For this review, use the dimensioned drawing (mm, ordinates from the lowest corner) and the shaded views. A direction names the side the tool comes from. Coordinates: 2 decimals unless noted, no trailing zeros. Order: outer loops, then holes, each group sorted by start corner. A loop starts at its lowest first (then second) coordinate and runs counter-clockwise, first axis right, second up. Notation, with made-up numbers: (64, 49) -> (87, 49) arc R17 cw to (87, 79) -> close; hole circle Ø8 at (30, 29.5). An arc over 180 degrees is marked (long way). Return JSON: item names as keys, results as strings. Group by question number.
Item 1: Insertion check: pin 1 (7 mm diameter, centred on y = 2.5, z = 3, fed in from -X); pin 2 (1 mm diameter, centred on x = 6, z = 7.5, fed in from -Y); pin 3 (2 mm diameter, centred on x = 13.5, z = 6.5, fed in from -Y). Each pin has a flat end and moves straight along its axis. Give the tip position at first contact, or say it passes through.
Item 2: Draft analysis for pull direction Y (two halves, no side actions). For the marked faces 1, 2 and 3, state which applies: +Y half, -Y half, draft (parallel to the pull), parting line (faces both ways), or undercut.
Item 3: Take a section at C-C (z = 8.5). Write out the cut boundary in (x, y).
Item 4: Take a section at A-A (x = 2.54). Write out the cut boundary in (y, z) (3 decimals).
Item 5: For line 1 along Z through (x, y) = (2.54, 12.25) (3 decimals); line 2 along Y through (x, z) = (4.5, 11.5); line 3 along Y through (x, z) = (14.25, 6.35) (3 decimals), list the stretches that pass through material, from the lowest coordinate up.
Item 6: Machinability: for the marked faces 4 and 5, which of the approach directions +Z, -Z, +X, -X, +Y, -Y give a long, thin tool a straight path to every point of the face, cutting with its end or side? Answer none if there is none.
Item 7: Take a section at D-D (z = 6.35). Write out the cut boundary in (x, y) (3 decimals), then the cut area to 3 significant figures.
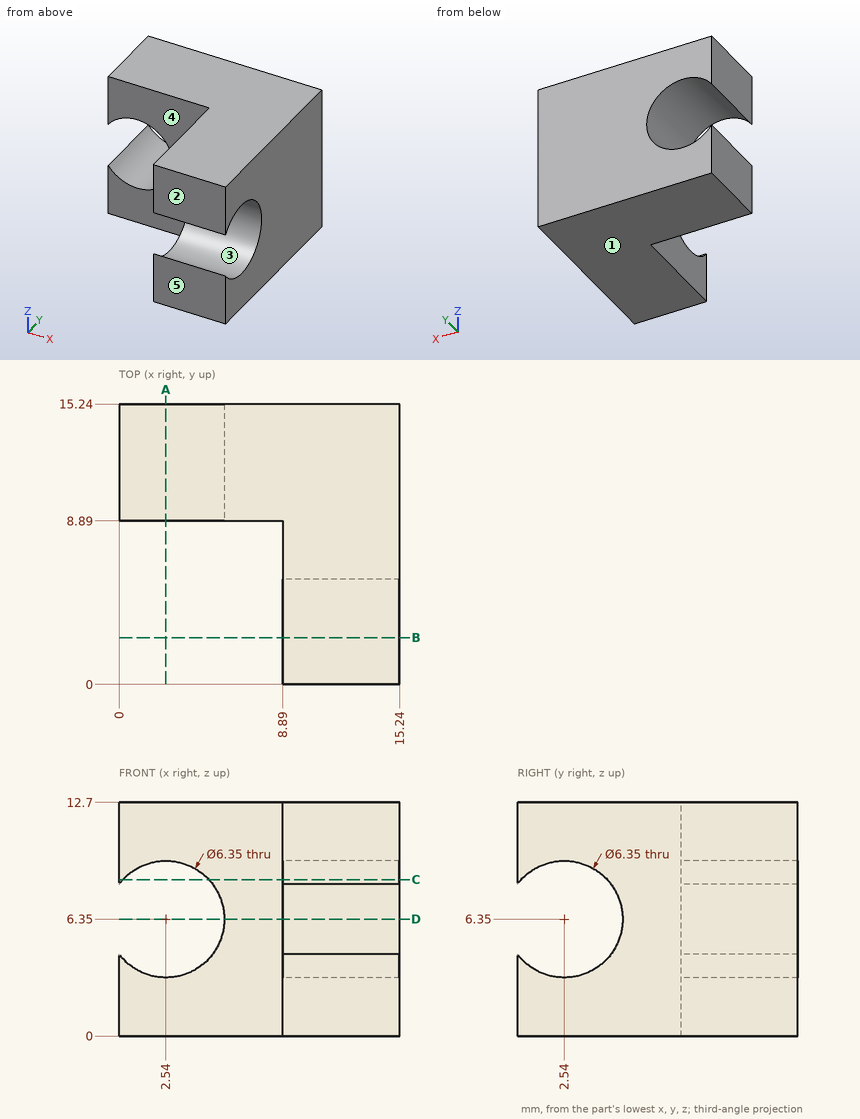
Findings below:
{
 "1": {"pin 1": "stops at x = 8.89", "pin 2": "stops at y = 8.89", "pin 3": "stops at y = 5.5"},
 "2": {"face 1": "draft", "face 2": "-Y half", "face 3": "undercut"},
 "3": {"outline": "(0, 8.89) -> (0.2, 8.89) -> (0.2, 15.24) -> (0, 15.24) -> close; (4.88, 8.89) -> (8.89, 8.89) -> (8.89, 4.88) -> (15.24, 4.88) -> (15.24, 15.24) -> (4.88, 15.24) -> close; (8.89, 0) -> (15.24, 0) -> (15.24, 0.2) -> (8.89, 0.2) -> close"},
 "4": {"outline": "(8.89, 0) -> (15.24, 0) -> (15.24, 3.175) -> (8.89, 3.175) -> close; (8.89, 9.525) -> (15.24, 9.525) -> (15.24, 12.7) -> (8.89, 12.7) -> close"},
 "5": {"line 1": "z = 0 to 3.175, 9.525 to 12.7", "line 2": "y = 8.89 to 15.24", "line 3": "y = 5.715 to 15.24"},
 "6": {"face 4": "+Z, -Z, -X, -Y", "face 5": "+Z, -Z, +X, -X, -Y"},
 "7": {"outline": "(5.715, 8.89) -> (8.89, 8.89) -> (8.89, 5.715) -> (15.24, 5.715) -> (15.24, 15.24) -> (5.715, 15.24) -> close", "area": "80.6 mm2"}
}
